Read the model definition and answer for the solid it produces. Units are mm, in the model's axes. A direction names the side the tool comes from. Round coordinates to 2 decimals unless told otherwise and drop trailing zeros. Write each loop counter-clockwise with the first axis right and the second up, starting at its lowest first coordinate (ties: lowest second). Pieces come first, ordered by that corner, then holes.
from build123d import *

# Parameters (mm, degrees)
SKETCH_1_W          = 160
SKETCH_1_H          = 20
EXTRUDE_1_DEPTH     = 5
EXTRUDE_3_DEPTH     = 100
SKETCH_5_W          = 12
SKETCH_5_H          = 15
EXTRUDE_4_DEPTH     = 105
SKETCH_6_W          = 74
SKETCH_6_H          = 15
EXTRUDE_5_DEPTH     = 5
SKETCH_7_W          = 160
SKETCH_7_H          = 35
EXTRUDE_6_DEPTH     = 5
EXTRUDE_7_DEPTH     = 5
SKETCH_9_R          = 2.75
CUT_EXTRUDE_1_DEPTH = 138.477270849
CHAMFER_1_SIZE      = 0.5
FILLET_1_R          = 10
EXTRUDE_8_DEPTH     = 5
FILLET_2_R          = 10


with BuildPart() as part:
    # 草图1 → 凸台-拉伸1 (new body)
    with BuildSketch(Plane(origin=(0, 0, 0), x_dir=(0, 0, -1), z_dir=(1, 0, 0))):
        with Locations((0, -5)):
            Rectangle(SKETCH_1_W, SKETCH_1_H)
    extrude(amount=EXTRUDE_1_DEPTH)

    # 草图3 → 凸台-拉伸3 (add)
    with BuildSketch(Plane(origin=(5, 0, 0), x_dir=(0, 0, -1), z_dir=(1, 0, 0))):
        Polygon((-6, 5), (6, 5), (6, -10), (20, -10), (20, -15), (-20, -15), (-20, -10), (-6, -10), align=None)
    extrude(amount=EXTRUDE_3_DEPTH)

    # 草图5 → 凸台-拉伸4 (add)
    with BuildSketch(Plane.ZY):
        with Locations((0, 12.5)):
            Rectangle(SKETCH_5_W, SKETCH_5_H)
    extrude(amount=-EXTRUDE_4_DEPTH)

    # 草图6 → 凸台-拉伸5 (add)
    with BuildSketch(Plane.ZY):
        with Locations((43, 12.5)):
            Rectangle(SKETCH_6_W, SKETCH_6_H)
        with Locations((-43, 12.5)):
            Rectangle(SKETCH_6_W, SKETCH_6_H)
    extrude(amount=-EXTRUDE_5_DEPTH)

    # 草图7 → 凸台-拉伸6 (add)
    with BuildSketch(Plane(origin=(105, 0, 0), x_dir=(0, 0, -1), z_dir=(1, 0, 0))):
        with Locations((0, 2.5)):
            Rectangle(SKETCH_7_W, SKETCH_7_H)
    extrude(amount=EXTRUDE_6_DEPTH)

    # 草图8 → 凸台-拉伸7 (add)
    with BuildSketch(Plane.XZ.offset(15)):
        Polygon((80, 20), (105, 65), (105, 20), align=None)
        Polygon((105, -20), (80, -20), (105, -65), align=None)
        Polygon((5, 20), (30, 20), (5, 65), align=None)
        Polygon((30, -20), (5, -65), (5, -20), align=None)
    extrude(amount=-EXTRUDE_7_DEPTH)

    # 草图9 → 切除-拉伸1 (cut, through all)
    with BuildSketch(Plane(origin=(110, 0, 0), x_dir=(0, 0, -1), z_dir=(1, 0, 0))):
        with Locations((45, 2.5)):
            Circle(SKETCH_9_R)
        with Locations(Location((-45, 2.5, 0), (0, 0, 180))):
            Circle(SKETCH_9_R)
    extrude(amount=-CUT_EXTRUDE_1_DEPTH, mode=Mode.SUBTRACT)

    # 倒角1
    chamfer_1_edges = [part.edges().sort_by_distance(p)[0] for p in [
        (105, 2.5, -42.25),
        (5, 2.5, -42.25),
        (0, 2.5, -42.25),
        (110, 2.5, -42.25),
        (105, 2.5, 42.25),
        (5, 2.5, 42.25),
        (0, 2.5, 42.25),
        (110, 2.5, 42.25),
    ]]
    chamfer(chamfer_1_edges, length=CHAMFER_1_SIZE)

    # 圆角1
    fillet_1_edges = [part.edges().sort_by_distance(p)[0] for p in [
        (107.5, -15, 80),
        (107.5, -15, -80),
        (2.5, -15, -80),
        (2.5, -15, 80),
    ]]
    fillet(fillet_1_edges, radius=FILLET_1_R)

    # 草图10 → 凸台-拉伸8 (add)
    with BuildSketch(Plane(origin=(0, 20, 0), x_dir=(1, 0, 0), z_dir=(0, 1, 0))):
        Polygon((5, 65), (5, 6), (105, 6), (105, 65), (80, 20), (30, 20), align=None)
        Polygon((5, -6), (5, -65), (30, -20), (80, -20), (105, -65), (105, -6), align=None)
    extrude(amount=-EXTRUDE_8_DEPTH)

    # 圆角2
    fillet_2_edges = [part.edges().sort_by_distance(p)[0] for p in [
        (2.5, 20, 80),
        (2.5, 20, -80),
        (107.5, 20, 80),
        (107.5, 20, -80),
    ]]
    fillet(fillet_2_edges, radius=FILLET_2_R)


solid = part.part
Q1. Section D-D (z = -45) is taken. State how many separate pieces and enclosed holes the cut face has, then the cut area to 3 significant figures.
Verdict:
separate pieces: 4
enclosed holes: 0
area: 516 mm2
Q2. Flat-ended cylindrical pins translate along their axes: pin 1 Ø1 at (x, y) = (34, 8) entering from +Z; pin 2 Ø4 at (x, y) = (54, -13.5) entering from +Z; pin 3 Ø12.5 at (x, y) = (71, 1.5) entering from -Z. Find the tip coordinate at first contact, or state that the pin passes through.
Verdict:
pin 1: stops at z = 6
pin 2: stops at z = 20
pin 3: stops at z = -6
Q3. Section C-C (x = 93) is taken. Determine the outline of the cut face in (y, z), then the cut area to 3 significant figures.
Verdict:
outline: (-15, -43.4) - (-10, -43.4) - (-10, -6) - (15, -6) - (15, -43.4) - (20, -43.4) - (20, 43.4) - (15, 43.4) - (15, 6) - (-10, 6) - (-10, 43.4) - (-15, 43.4) - close
area: 1,170 mm2
Q4. Section B-B (z = 33.5) is taken. Determine the outline of the cut face in (x, y).
Verdict:
outline: (0, -15) - (22.5, -15) - (22.5, -10) - (5, -10) - (5, 15) - (22.5, 15) - (22.5, 20) - (0, 20) - close; (87.5, -15) - (110, -15) - (110, 20) - (87.5, 20) - (87.5, 15) - (105, 15) - (105, -10) - (87.5, -10) - close
Q5. Which of the six approach directions +Z, -Z, +X, -X, +Y, -Y give full straight-line access (tool end or side, diameter ignored) to faces 5 (the flat face through (92.68, 17.54, -42.82)), 6 (the flat face through (105, 7, -42)), 7 (the flat face through (17.675, -12.535, 42.185)), 8 (the cylindrical face through (107.54, 17.15, -76.99))?
Verdict:
face 5: -Z, +Y, -Y
face 6: -Z
face 7: +Z, +Y, -Y
face 8: -Z, +X, -X, +Y
Q6. Section A-A (z = -17.5) is taken. Determine the outline of the cut face in (x, y).
Verdict:
outline: (0, -15) - (110, -15) - (110, 20) - (0, 20) - close; hole (5, -10) - (105, -10) - (105, 15) - (5, 15) - close
Q7. Determine the mould class of faces 1 (the flat face through (54, -10, -15)), 2 (the flat face through (92.32, -12.54, -42.18)), 3 (the flat face through (54, 2, -6)), 4 (the cylindrical face through (2.54, 17.15, -76.99)) for opening direction Y: pulls with the +Y half, pulls with the -Y half, needs draft (parallel to the pull), parting line crosses it, or undercut.
Verdict:
face 1: undercut
face 2: needs draft
face 3: undercut
face 4: pulls with the +Y half
Q8. Straight lines are drawn through the part: probe 1 along Z at (x, y) = (106, 2); probe 2 along Y at (x, z) = (2.15, -45); probe 3 along X at (y, z) = (5, -31.5). For each, find the intervals that lie inside material, in ascending order.
Verdict:
probe 1: z = -80 to -47.7, -42.3 to 42.3, 47.7 to 80
probe 2: y = -15 to -0.25, 5.25 to 20
probe 3: x = 0 to 5, 105 to 110
